Input: part model. Units: mm. Frame: model coordinates. A direction names the side the tool comes from. Coordinates: 2 decimals unless noted, no trailing zeros. Loops run counter-clockwise (first coordinate to the right, second up) from the corner with the lowest first, then second, coordinate; pieces in that order, holes last. Notation, with made-up numbers: (40, 27) - (71, 27) arc R15 ccw to (71, 51) - close; hole circle Ø1 at (89, -0.5). An arc over 180 degrees is marked (long way). Use a Markdown table: item, result. Add a question column.
1. Draft query along X for faces 1 (the face through (0, 11.4, 0)), 2 (the face through (-2.86, 6.68, 5.5)), 3 (the face through (0, 0, 0)). Return one class per face: released by +X, released by -X, zero draft, split by the parting line, or undercut.
2. Ray query, L1, parallel to Y at x = -0.25, z = 6.25; L2, parallel to Y at x = -1.75, z = 5.5; L3, parallel to Z at x = 1.5, y = 7. Return the intervals inside material, ascending. Write a range as [from, to].
3. Access query for faces 4 (the face through (1.5, 0.49, -0.07)), 5 (the face through (0.9, 1.25, -6.84)), 6 (the face through (-5, 1.5, -4)). Directions: +Z, -Z, +X, -X, +Y, -Y. A direction counts if a zero-diameter tool reaches every point of the face in a straight line with its end or side. Return the directions, or none.
4. Section query A-A on z = 5.75. Return the cut outline in (x, y).
5. Section query B-B on y = 7.25. Return the cut outline in (x, z).
6. Contact query for flat-ended pins moving along their axis: P1, Ø1.5, axis at y = 4.5, z = -1, coming from the +X side; P2, Ø2, axis at x = 4.5, z = 1.5, coming from the -Y side; P3, Ø1.5, axis at x = -5, y = 8.5, coming from the +Z side. Output: stop coordinate, or through.
```python
from build123d import *


with BuildPart() as part:
    # Sketch 183 → Revolve1 (revolve)
    with BuildSketch(Plane.XY):
        with BuildLine():
            Line((-5.2, 12), (-6.2, 12))
            Line((-6.2, 12), (-6.2, 1.5))
            Line((-6.2, 1.5), (-6.9, 1.5))
            Line((-6.9, 1.5), (-6.9, 1))
            Line((-6.9, 1), (-6.2, 1))
            Line((-6.2, 1), (-1.5, 1))
            Line((-1.5, 1), (-1.5, 0))
            Line((-1.5, 0), (0, 0))
            Line((0, 0), (0, 11.400347218))
            Line((0, 11.400347218), (-1, 11.400347218))
            ThreePointArc((-1, 11.400347218), (-3.071763766, 11.544109643), (-5.103815293, 11.972641231))
            Line((-5.103815293, 11.972641231), (-5.2, 12))
        make_face()
    revolve(axis=Axis((0, 11.400347218, 0), (0, -1, 0)))


solid = part.part
```
Resolved:
| question | item | result |
|---|---|---|
| 1 | face 1 | undercut |
| 1 | face 2 | split by the parting line |
| 1 | face 3 | zero draft |
| 2 | L1 | [1, 1.5] |
| 2 | L2 | [1, 12] |
| 2 | L3 | [-6.02, 6.02] |
| 3 | face 4 | -Y |
| 3 | face 5 | +Y, -Y |
| 3 | face 6 | +Y |
| 4 | outline | (-3.81, 1) - (3.81, 1) - (3.81, 1.5) - (2.32, 1.5) - (2.32, 12) - (-2.32, 12) - (-2.32, 1.5) - (-3.81, 1.5) - close |
| 5 | outline | circle Ø12.4 at (0, 0) |
| 6 | P1 | x = 6.19 |
| 6 | P2 | y = 1 |
| 6 | P3 | z = 4.51 |
